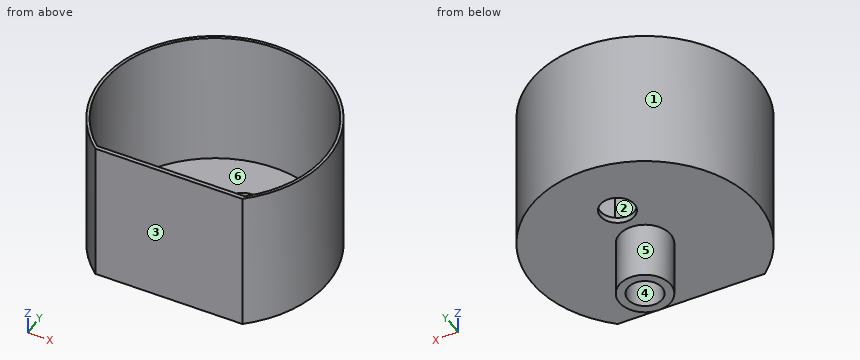
from build123d import *

# Parameters (mm, degrees)
BOSS_EXTRUDE1_DEPTH = 50
BOSS_EXTRUDE2_DEPTH = 2
SKETCH3_R           = 6
CUT_EXTRUDE1_DEPTH  = 2
SKETCH4_R           = 6
CUT_EXTRUDE2_DEPTH  = 2
BOSS_EXTRUDE3_START = 20
SKETCH5_R           = 9
SKETCH5_R_2         = 6
BOSS_EXTRUDE3_DEPTH = 20


with BuildPart() as part:
    # Sketch1 → Boss-Extrude1 (new body)
    with BuildSketch(Plane.XY):
        with BuildLine():
            Line((-25.576977383, -30.100967226), (25.576977383, -30.100967226))
            ThreePointArc((25.576977383, -30.100967226), (0, 39.5), (-25.576977383, -30.100967226))
        make_face()
        with BuildLine():
            Line((-25.687078778, -28.677935488), (25.687078778, -28.677935488))
            ThreePointArc((25.687078778, -28.677935488), (0, 38.5), (-25.687078778, -28.677935488))
        make_face(mode=Mode.SUBTRACT)
    extrude(amount=BOSS_EXTRUDE1_DEPTH)

    # Sketch2 → Boss-Extrude2 (add)
    with BuildSketch(Plane(origin=(0, 0, 0), x_dir=(-1, 0, 0), z_dir=(0, 0, -1))):
        with BuildLine():
            Line((25.687078778, -28.677935488), (-25.687078778, -28.677935488))
            ThreePointArc((-25.687078778, -28.677935488), (0, 38.5), (25.687078778, -28.677935488))
        make_face()
    extrude(amount=-BOSS_EXTRUDE2_DEPTH)

    # Sketch3 → Cut-Extrude1 (cut)
    with BuildSketch(Plane(origin=(0, 0, 0), x_dir=(-1, 0, 0), z_dir=(0, 0, -1))):
        Circle(SKETCH3_R)
    extrude(amount=-CUT_EXTRUDE1_DEPTH, mode=Mode.SUBTRACT)

    # Sketch4 → Cut-Extrude2 (cut)
    with BuildSketch(Plane(origin=(0, 0, 0), x_dir=(-1, 0, 0), z_dir=(0, 0, -1))):
        with Locations((0, 18)):
            Circle(SKETCH4_R)
    extrude(amount=-CUT_EXTRUDE2_DEPTH, mode=Mode.SUBTRACT)

    # Sketch5 → Boss-Extrude3 (add)
    with BuildSketch(Plane(origin=(0, 0, 0), x_dir=(-1, 0, 0), z_dir=(0, 0, -1)).offset(BOSS_EXTRUDE3_START)):
        with Locations(Location((0, 0, 0), (0, 0, 180))):
            Circle(SKETCH5_R)
        Circle(SKETCH5_R_2, mode=Mode.SUBTRACT)
    extrude(amount=-BOSS_EXTRUDE3_DEPTH)


solid = part.part
Can you work these out from the model? Positions are in its coordinate system, mm. Face numbers are marked on the shaded views. A direction names the side the tool comes from. Coordinates: 2 decimals unless noted, no trailing zeros. Write each loop counter-clockwise with the first axis right and the second up, starting at its lowest first coordinate (ties: lowest second). Pieces come first, ordered by that corner, then holes.
Q1. Imagine slicing it at A-A, the plane x = 0. List the corners of the cut face in (y, z) for me, plus the area to 3 significant figures.
Results found:
outline: (-30.1, 0) - (-9, 0) - (-9, -20) - (-6, -20) - (-6, 2) - (-28.68, 2) - (-28.68, 50) - (-30.1, 50) - close; (6, -20) - (9, -20) - (9, 0) - (12, 0) - (12, 2) - (6, 2) - close; (24, 0) - (39.5, 0) - (39.5, 50) - (38.5, 50) - (38.5, 2) - (24, 2) - close
area: 328 mm2
Q2. If we mould it in two halves opening along X, with no side actions, what happens to the marked faces 1, 2 and 3? For each: +X half, -X half, draft (parallel to the pull), parting line (faces both ways), or undercut.
Results found:
face 1: parting line
face 2: undercut
face 3: draft
Q3. Imagine slicing it at D-D, the plane z = -3.5. List the corners of the cut face in (x, y) for me, plus the area to 3 significant figures.
Results found:
outline: circle Ø18 at (0, 0); hole circle Ø12 at (0, 0)
area: 141 mm2
Q4. For P1, Ø5, axis at x = -20.5, y = -10, coming from the +Z side; P2, Ø1.5, axis at y = -13, z = 23.5, coming from the -X side; P3, Ø9.5, axis at x = 0, y = 0, coming from the +Z side; P4, Ø3, axis at x = 30, y = -16.5, coming from the -Z side, each with a flat end and sliding along its axis, tell me the tip position at first contact or that it passes through.
Results found:
P1: stops at z = 2
P2: stops at x = -37.55
P3: passes through
P4: stops at z = 0
Q5. Imagine slicing it at C-C, the plane x = 19. List the corners of the cut face in (y, z) for me.
Results found:
outline: (-30.1, 0) - (34.63, 0) - (34.63, 50) - (33.49, 50) - (33.49, 2) - (-28.68, 2) - (-28.68, 50) - (-30.1, 50) - close
Q6. Which directions (+Z, -Z, +X, -X, +Y, -Y) give clear straight access to the entire face, cutting with the end or side of a thin tool? Please do the marked faces 4, 5 and 6.
Results found:
face 4: +Z, -Z
face 5: -Z
face 6: +Z
Q7. Please list where these lines run through material, in increasing order: L1, parallel to Y at x = 0, z = 0.9; L2, parallel to Z at x = 19.5, y = 5; L3, parallel to X at y = 0, z = 21.
Results found:
L1: y = -30.1 to -6, 6 to 12, 24 to 39.5
L2: z = 0 to 2
L3: x = -39.5 to -38.5, 38.5 to 39.5
Q8. Imagine slicing it at B-B, the plane y = 0. List the corners of the cut face in (x, z) for me.
Results found:
outline: (-39.5, 0) - (-9, 0) - (-9, -20) - (-6, -20) - (-6, 2) - (-38.5, 2) - (-38.5, 50) - (-39.5, 50) - close; (6, -20) - (9, -20) - (9, 0) - (39.5, 0) - (39.5, 50) - (38.5, 50) - (38.5, 2) - (6, 2) - close
